Check sheet for the modelled part. Datum: model origin and axes. Units: mm. A direction names the side the tool comes from. Give positions to 0.01 mm unless a question says otherwise; leave off trailing zeros. Order: outer loops, then holes, each group sorted by start corner. A loop starts at its lowest first (then second) coordinate and runs counter-clockwise, first axis right, second up.
Autodesk Inventor part; units mm, degrees
ref_plane "YZ Plane" through (0, 0, 0) normal (1, 0, 0) x (0, 1, 0)
ref_plane "XZ Plane" through (0, 0, 0) normal (0, 1, 0) x (-1, 0, 0)
ref_plane "XY Plane" through (0, 0, 0) normal (0, 0, 1) x (1, 0, 0)
sketch "スケッチ1" plane through (0, 0, 0) normal (0, 1, 0) x (-1, 0, 0)
  line L0 (0, 0) -> (23, 0)
  line L1 (23, 0) -> (23, -12.2)
  line L2 (23, -12.2) -> (0, -12.2)
  line L3 (0, -12.2) -> (0, 0)
  dimension "d0" = 23
  dimension "d1" = 12.2
extrude "押し出し1" add sketch "スケッチ1" along normal blind 27
sketch "スケッチ2" plane through (0, 0, 0) normal (1, 0, 0) x (0, 0, -1)
  line L0 (0, 0) -> (0, 16)
  line L1 (0, 0) -> (0, 27)
  line L2 (0, 16) -> (12.2, 16)
  line L3 (12.2, 0) -> (12.2, 27)
  line L4 (0, 16) -> (0, 19)
  line L5 (0, 19) -> (12.2, 19)
  line L6 (12.2, 19) -> (12.2, 16)
  dimension "d4" = 16
  dimension "d5" = 3
extrude "押し出し2" add sketch "スケッチ2" along normal blind 4
sketch "スケッチ3" plane through (-23, 0, -12.2) normal (-1, 0, 0) x (0, 0, 1)
  line L0 (0, 0) -> (0, 16.2076)
  line L1 (0, 16.2076) -> (12.2, 16.2076)
  line L2 (12.2, 16.2076) -> (12.2, 19.2076)
  line L3 (12.2, 19.2076) -> (0, 19.2076)
  line L4 (0, 0) -> (0, 27)
  line L5 (0, 19.2076) -> (0, 16.2076)
  point P0 (12.2, 0)
  dimension "d8" = 3
extrude "押し出し3" add sketch "スケッチ3" along normal blind 4
hole "穴2" at (-25, 19.2076, -6.1) direction (0, -1, 0) diameter 2 end through all
hole "穴3" at (2, 19, -6.1) direction (0, -1, 0) diameter 2 end through all
properties part number "サーボ"
1) Draft check along Z on faces 1 (the face through (-24.11, 17.69, -5.64)), 2 (the face through (-11, 0, -6)), 3 (the face through (-11, 13, 0)), 4 (the face through (1.7, 17.479, -5.146)). Enter one of: +Z half, -Z half, draft (parallel to the pull), parting line (faces both ways), or undercut.
Recorded:
face 1: undercut
face 2: draft
face 3: +Z half
face 4: undercut
2) Section check C-C, the plane z = -2.75. Record the cut outline in (x, y).
Recorded:
outline: (-27, 16.21) - (-23, 16.21) - (-23, 0) - (0, 0) - (0, 16) - (4, 16) - (4, 19) - (0, 19) - (0, 27) - (-23, 27) - (-23, 19.21) - (-27, 19.21) - close
3) Section check B-B, the plane z = -6.1. Record the cut outline in (x, y), then the cut area to 3 significant figures.
Recorded:
outline: (-27, 16.21) - (-26, 16.21) - (-26, 19.21) - (-27, 19.21) - close; (-24, 16.21) - (-23, 16.21) - (-23, 0) - (0, 0) - (0, 16) - (1, 16) - (1, 19) - (0, 19) - (0, 27) - (-23, 27) - (-23, 19.21) - (-24, 19.21) - close; (3, 16) - (4, 16) - (4, 19) - (3, 19) - close
area: 633 mm2
4) Depth check by flat-ended pin: pin 1 Ø4 at (y, z) = (22.5, -6.5) entering from -X; pin 2 Ø1.2 at (x, z) = (2.5, -4.5) entering from -Y; pin 3 Ø3 at (x, z) = (-25, -6.1) entering from +Y; pin 4 Ø5 at (x, z) = (-5.5, -6) entering from -Y. Enter the tip coordinate at first touch or a pass-through.
Recorded:
pin 1: stops at x = -23
pin 2: stops at y = 16
pin 3: stops at y = 19.21
pin 4: stops at y = 0
5) Set-up check for faces 5 (the face through (3.3, 16, -6)), 6 (the face through (-26.3, 19.208, -6)), 7 (the face through (3.3, 19, -6)): record each of +Z, -Z, +X, -X, +Y, -Y from which the full face is reachable in a straight line by a thin tool's end or side.
Recorded:
face 5: +Z, -Z, +X, -Y
face 6: +Z, -Z, -X, +Y
face 7: +Z, -Z, +X, +Y
6) Section check D-D, the plane y = 13.25. Record the cut outline in (x, z).
Recorded:
outline: (-23, -12.2) - (0, -12.2) - (0, 0) - (-23, 0) - close
7) Material ranges on L1, parallel to X at y = 17.95, z = -6.1; L2, parallel to Z at x = -25, y = 16.9; L3, parallel to Y at x = 1.5, z = -9, recorded low to high.
Recorded:
L1: x = -27 to -26, -24 to 1, 3 to 4
L2: z = -12.2 to -7.1, -5.1 to 0
L3: y = 16 to 19
8) Section check A-A, the plane x = -25. Record the cut outline in (y, z).
Recorded:
outline: (16.21, -12.2) - (19.21, -12.2) - (19.21, -7.1) - (16.21, -7.1) - close; (16.21, -5.1) - (19.21, -5.1) - (19.21, 0) - (16.21, 0) - close
